```python
from build123d import *

# Parameters (mm, degrees)
SKETCH1_W           = 20
SKETCH1_H           = 20
BOSS_EXTRUDE1_DEPTH = 500
SKETCH2_W           = 19
SKETCH2_H           = 19
CUT_EXTRUDE1_DEPTH  = 501.199960016
SKETCH3_R           = 2
CUT_EXTRUDE2_DEPTH  = 20
SKETCH5_R           = 4
CUT_EXTRUDE3_DEPTH  = 20


with BuildPart() as part:
    # Sketch1 → Boss-Extrude1 (new body)
    with BuildSketch(Plane.XY):
        Rectangle(SKETCH1_W, SKETCH1_H)
    extrude(amount=BOSS_EXTRUDE1_DEPTH)

    # Sketch2 → Cut-Extrude1 (cut, through all)
    with BuildSketch(Plane(origin=(0, 0, 0), x_dir=(-1, 0, 0), z_dir=(0, 0, -1))):
        Rectangle(SKETCH2_W, SKETCH2_H)
    extrude(amount=-CUT_EXTRUDE1_DEPTH, mode=Mode.SUBTRACT)

    # Sketch3 → Cut-Extrude2 (cut)
    with BuildSketch(Plane(origin=(0, 10, 0), x_dir=(1, 0, 0), z_dir=(0, 1, 0))):
        with Locations(Location((0, -60, 0), (0, 0, 270))):
            Circle(SKETCH3_R)
    extrude(amount=-CUT_EXTRUDE2_DEPTH, mode=Mode.SUBTRACT)

    # Sketch5 → Cut-Extrude3 (cut)
    with BuildSketch(Plane.ZY.offset(10)):
        with Locations((450, 0)):
            Circle(SKETCH5_R)
    extrude(amount=-CUT_EXTRUDE3_DEPTH, mode=Mode.SUBTRACT)


solid = part.part
```
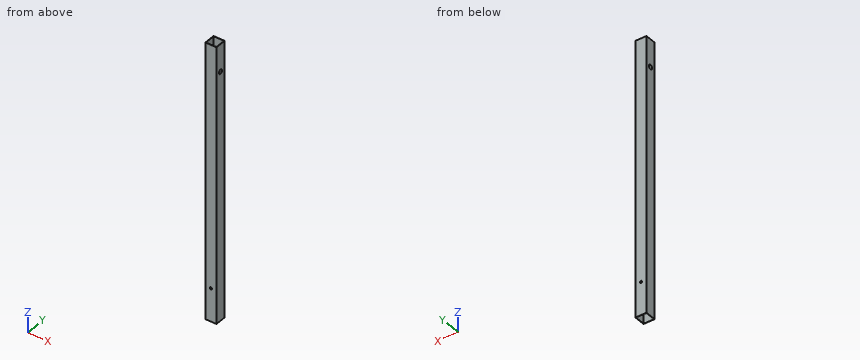
The listing builds one solid part. Answer for the finished solid, in the listing's coordinates (mm). Give positions to 0.01 mm unless a question says otherwise; leave off trailing zeros. Order: outer loops, then holes, each group sorted by start corner. A loop starts at its lowest first (then second) coordinate and runs counter-clockwise, first axis right, second up.
1) Find section B-B on x = 5.25. Write down the section's boundary in (y, z).
Reported:
outline: (-10, 0) - (-9.5, 0) - (-9.5, 500) - (-10, 500) - close; (9.5, 0) - (10, 0) - (10, 500) - (9.5, 500) - close
2) Consider line 1 along Y through (x, z) = (1, 449); line 2 along Y through (x, z) = (-9.7, 450). Determine where each line is inside the solid, lowest interval first.
Reported:
line 1: y = -10 to -9.5, 9.5 to 10
line 2: y = -10 to -4, 4 to 10
3) Given P1, Ø10, axis at x = -6.5, y = -3, coming from the -Z side; P2, Ø3, axis at x = 7, y = 5, coming from the +Z side, each flat-ended and moving along its own axis, determine where each tip first touches the part or whether it passes through.
Reported:
P1: stops at z = 0
P2: passes through
4) Find section A-A on z = 214. Write down the section's boundary in (x, y), then the cut area to 3 significant figures.
Reported:
outline: (-10, -10) - (10, -10) - (10, 10) - (-10, 10) - close; hole (-9.5, -9.5) - (9.5, -9.5) - (9.5, 9.5) - (-9.5, 9.5) - close
area: 39.0 mm2
5) Find section C-C on y = 0. Write down the section's boundary in (x, z).
Reported:
outline: (-10, 0) - (-9.5, 0) - (-9.5, 446) - (-10, 446) - close; (-10, 454) - (-9.5, 454) - (-9.5, 500) - (-10, 500) - close; (9.5, 0) - (10, 0) - (10, 446) - (9.5, 446) - close; (9.5, 454) - (10, 454) - (10, 500) - (9.5, 500) - close
